The model under review builds one solid part; all positions refer to its coordinate system, in mm. Face numbers are marked on the shaded views. Round coordinates to 2 decimals unless told otherwise and drop trailing zeros. Answer as a JSON object with one key per item and string values. Group by question number.
1) The part is to be moulded in two halves that separate along X. For the marked faces 1, 2 and 3, say which applies: +X half, -X half, draft (parallel to the pull), parting line (faces both ways), or undercut.
2) To check wall thickness, follow line 1 (X direction, y = -5.5, z = 20.5); line 2 (X direction, y = -24, z = 80.5); line 3 (Y direction, x = -27.5, z = 12). State the ranges of each line that lie inside material, in increasing order.
3) Insertion check: pin 1 Ø1.5 at (x, y) = (66, -76.5) entering from +Z. The pin has a flat end and moves straight along its axis. Give the tip position at first contact, or say it passes through.
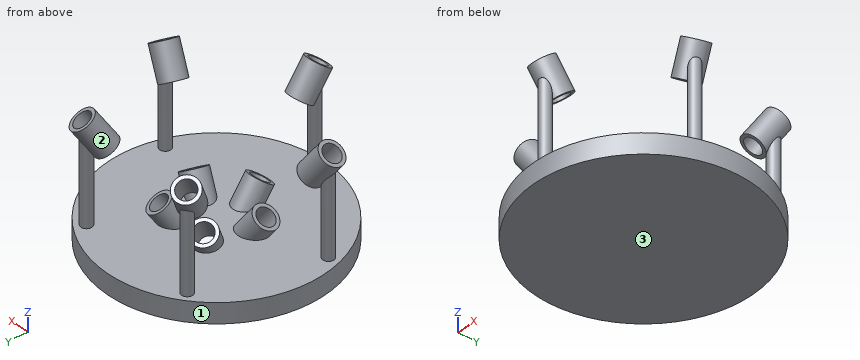
```python
from build123d import *

# Parameters (mm, degrees)
SKETCH1_R            = 98.5
BOSS_EXTRUDE1_DEPTH  = 9
SWEEP2_PROFILE_R     = 11
SKETCH65_R           = 5
BOSS_EXTRUDE2_DEPTH  = 96
CUT_SWEEP1_PROFILE_R = 8
CUT_SWEEP8_PROFILE_R = 11
CUT_SWEEP7_PROFILE_R = 2.5
CIRPATTERN1_COUNT    = 5


with BuildPart() as part:
    # Sketch1 → Boss-Extrude1 (new, symmetric)
    with BuildSketch(Plane.XY):
        Circle(SKETCH1_R)
    extrude(amount=BOSS_EXTRUDE1_DEPTH, both=True)

    # Sweep2: sweep along a path in Sketch3
    with BuildLine(Plane(origin=(0, 0, 0), x_dir=(0, 0, -1), z_dir=(1, 0, 0))) as sweep2_path:
        Line((0, -22), (-97.537036334, -91.903694775))
    # Sweep2 profile (on start of the path) → Sweep2 (sweep)
    with BuildSketch(Plane(origin=(0, -22, 0), x_dir=(0, 0.8128086361148117, 0.5825307897932775), z_dir=(0, -0.5825307897932775, 0.8128086361148117))):
        Circle(SWEEP2_PROFILE_R)
    sweep2 = sweep(path=sweep2_path.line)

    # Sketch65 → Boss-Extrude2 (add)
    with BuildSketch(Plane.XY):
        with Locations(Location((0, -89, 0), (0, 0, 90))):
            Circle(SKETCH65_R)
    boss_extrude2 = extrude(amount=BOSS_EXTRUDE2_DEPTH)

    # Cut-Sweep1: sweep along a path in Sketch3_2
    with BuildLine(Plane(origin=(0, 0, 0), x_dir=(0, 0, -1), z_dir=(1, 0, 0))) as cut_sweep1_path:
        Line((0, -22), (-97.537036334, -91.903694775))
    # Cut-Sweep1 profile (on start of the path) → Cut-Sweep1 (sweep, cut)
    with BuildSketch(Plane(origin=(0, -22, 0), x_dir=(0, 0.8128086361148117, 0.5825307897932775), z_dir=(0, -0.5825307897932775, 0.8128086361148117))):
        Circle(CUT_SWEEP1_PROFILE_R)
    cut_sweep1 = sweep(path=cut_sweep1_path.line, mode=Mode.SUBTRACT)

    # Cut-Sweep8: sweep along a path in Sketch534
    with BuildLine(Plane(origin=(0, 0, 0), x_dir=(0, 0, -1), z_dir=(1, 0, 0))) as cut_sweep8_path:
        Line((-24.237328538, -39.370620228), (-74.016413707, -75.046729597))
    # Cut-Sweep8 profile (on start of the path) → Cut-Sweep8 (sweep, cut)
    with BuildSketch(Plane(origin=(0, -39.370620228, 24.237328538), x_dir=(0, 0.8128086361148117, 0.5825307897932777), z_dir=(0, -0.5825307897932777, 0.8128086361148117))):
        Circle(CUT_SWEEP8_PROFILE_R)
    cut_sweep8 = sweep(path=cut_sweep8_path.line, mode=Mode.SUBTRACT)

    # Cut-Sweep7: sweep along a path in Sketch199
    with BuildLine(Plane(origin=(0, 0, 0), x_dir=(0, 0, -1), z_dir=(1, 0, 0))) as cut_sweep7_path:
        Line((5.317627658, -21.308382404), (-9, -28.450198577))
    # Cut-Sweep7 profile (on start of the path) → Cut-Sweep7 (sweep, cut)
    with BuildSketch(Plane(origin=(0, -21.308382404, -5.317627658), x_dir=(0, 0.89485172861867, 0.44636351081621606), z_dir=(0, -0.44636351081621606, 0.89485172861867))):
        Circle(CUT_SWEEP7_PROFILE_R)
    cut_sweep7 = sweep(path=cut_sweep7_path.line, mode=Mode.SUBTRACT)

    # CirPattern1: Sweep2, Boss-Extrude2, Cut-Sweep1, Cut-Sweep8, Cut-Sweep7 ×5 about axis
    cirpattern1_axis = Axis((0, 0, 0), (0, 0, 1))
    add([sweep2.rotate(cirpattern1_axis, i * 360 / CIRPATTERN1_COUNT) for i in range(1, CIRPATTERN1_COUNT)])
    add([boss_extrude2.rotate(cirpattern1_axis, i * 360 / CIRPATTERN1_COUNT) for i in range(1, CIRPATTERN1_COUNT)])
    add([cut_sweep1.rotate(cirpattern1_axis, i * 360 / CIRPATTERN1_COUNT) for i in range(1, CIRPATTERN1_COUNT)], mode=Mode.SUBTRACT)
    add([cut_sweep8.rotate(cirpattern1_axis, i * 360 / CIRPATTERN1_COUNT) for i in range(1, CIRPATTERN1_COUNT)], mode=Mode.SUBTRACT)
    add([cut_sweep7.rotate(cirpattern1_axis, i * 360 / CIRPATTERN1_COUNT) for i in range(1, CIRPATTERN1_COUNT)], mode=Mode.SUBTRACT)


solid = part.part
```
Results list:
{
 "1": {"face 1": "parting line", "face 2": "undercut", "face 3": "draft"},
 "2": {"line 1": "-45.09 to -40.8, -27.31 to -22.76, 22.76 to 27.31, 40.8 to 45.09", "line 2": "-88.9 to -85.28, -66.12 to -62.51, 62.51 to 66.12, 85.28 to 88.9", "line 3": "-20.39 to -17.31, -1.27 to 1.81, 19.2 to 34.26"},
 "3": {"pin 1": "through"}
}
